```python
from build123d import *

# Parameters (mm, degrees)
SKETCH1_R               = 67.31
SKETCH1_R_2             = 54.61
BOSS_EXTRUDE1_DEPTH     = 57.15
CUT_EXTRUDE1_DEPTH      = 161.994729727
CUT_EXTRUDE1_DEPTH_BACK = 161.994729727
SKETCH2_R               = 1.2065
SKETCH3_R               = 1.2065
CUT_EXTRUDE2_DEPTH      = 171.985259226
CUT_EXTRUDE3_START      = -50.8
CUT_EXTRUDE3_DEPTH      = 50.8
SKETCH5_W               = 12.7
SKETCH5_H               = 152.473493429
CUT_EXTRUDE4_DEPTH      = 50.8
CUT_EXTRUDE5_START      = -19.05
CUT_EXTRUDE5_DEPTH      = 19.05
CUT_EXTRUDE6_START      = -19.05
CUT_EXTRUDE6_DEPTH      = 19.05
FILLET1_START           = 53
FILLET1_DEPTH           = 15
FILLET1_2_DEPTH         = 15
FILLET1_START_2         = -67.31
FILLET1_3_DEPTH         = 14.31
CUT_EXTRUDE7_START      = -19.05
CUT_EXTRUDE7_DEPTH      = 19.05


with BuildPart() as part:
    # Sketch1 → Boss-Extrude1 (new body)
    with BuildSketch(Plane(origin=(0, 0, 0), x_dir=(1, 0, 0), z_dir=(0, 1, 0))):
        with Locations(Location((0, 0, 0), (0, 0, 270))):
            Circle(SKETCH1_R)
        with Locations(Location((0, 0, 0), (0, 0, 270))):
            Circle(SKETCH1_R_2, mode=Mode.SUBTRACT)
    extrude(amount=BOSS_EXTRUDE1_DEPTH)

    # Sketch2 → Cut-Extrude1 (cut, two sides: drawn at the far end of the back side and taken through both)
    with BuildSketch(Plane.XY.offset(67.31).offset(-CUT_EXTRUDE1_DEPTH_BACK)):
        Polygon((-5.08, 51.435), (-6.35, 52.705), (-6.35, 50.165), align=None)
        Polygon((-6.35, 52.705), (-6.35, 57.15), (-19.05, 57.15), (-19.05, 25.0825), (-6.35, 25.0825), (-6.35, 50.165), align=None)
        Polygon((5.08, 51.435), (6.35, 50.165), (6.35, 52.705), align=None)
        Polygon((6.35, 50.165), (6.35, 25.0825), (19.05, 25.0825), (19.05, 57.15), (6.35, 57.15), (6.35, 52.705), align=None)
        with Locations((0, 51.435)):
            Circle(SKETCH2_R)
        with Locations((0, 28.575)):
            Circle(SKETCH2_R)
        with Locations((0, 5.715)):
            Circle(SKETCH2_R)
    extrude(amount=CUT_EXTRUDE1_DEPTH + CUT_EXTRUDE1_DEPTH_BACK, mode=Mode.SUBTRACT)

    # Sketch3 → Cut-Extrude2 (cut, through all)
    with BuildSketch(Plane(origin=(-58.292169929, 0, -33.655), x_dir=(0, -1, 0), z_dir=(-0.8660254037844364, 0, -0.5000000000000041))):
        with Locations(Location((-28.575, 0, 0), (0, 0, 90))):
            Circle(SKETCH3_R)
    cut_extrude2 = extrude(amount=-CUT_EXTRUDE2_DEPTH, mode=Mode.SUBTRACT)

    # Mirror1: Cut-Extrude2 across plane
    add(cut_extrude2.mirror(Plane(origin=(0, 0, 0), x_dir=(0, 0, 1), z_dir=(1, 0, 0))), mode=Mode.SUBTRACT)

    # Cut-Extrude3: read off the stored shape, not the designer's step
    # Cut-Extrude3 outline → Cut-Extrude3 (cut)
    with BuildSketch(Plane(origin=(0, 57.15, 0), x_dir=(1, 0, 0), z_dir=(0, 1, 0)).offset(CUT_EXTRUDE3_START)):
        with BuildLine():
            ThreePointArc((-6.35, -67.009802268), (0, -67.31), (6.35, -67.009802268))
            Line((6.35, -67.009802268), (-6.35, -67.009802268))
        make_face()
        with BuildLine():
            Line((6.35, -54.23955752), (6.35, -67.009802268))
            ThreePointArc((6.35, -67.009802268), (57.986556059, -34.178873833), (61.701920082, 26.898125551))
            Line((61.701920082, 26.898125551), (50.616947204, 20.498213476))
            ThreePointArc((50.616947204, 20.498213476), (46.986613751, -27.830023862), (6.35, -54.23955752))
        make_face()
        with BuildLine():
            Line((-6.35, -67.009802268), (-6.35, -54.23955752))
            ThreePointArc((-6.35, -54.23955752), (-46.986613751, -27.830023862), (-50.616947204, 20.498213476))
            Line((-50.616947204, 20.498213476), (-61.701920082, 26.898125551))
            ThreePointArc((-61.701920082, 26.898125551), (-57.986556059, -34.178873833), (-6.35, -67.009802268))
        make_face()
        with BuildLine():
            Line((54.145420082, 39.986367478), (61.701920082, 26.898125551))
            ThreePointArc((61.701920082, 26.898125551), (58.292169929, 33.655), (54.145420082, 39.986367478))
        make_face()
        with BuildLine():
            Line((-54.145420082, 39.986367478), (-43.060447204, 33.586455403))
            ThreePointArc((-43.060447204, 33.586455403), (0, 54.61), (43.060447204, 33.586455403))
            Line((43.060447204, 33.586455403), (54.145420082, 39.986367478))
            ThreePointArc((54.145420082, 39.986367478), (0, 67.31), (-54.145420082, 39.986367478))
        make_face()
    extrude(amount=CUT_EXTRUDE3_DEPTH, mode=Mode.SUBTRACT)

    # Sketch5 → Cut-Extrude4 (cut)
    with BuildSketch(Plane(origin=(0, 6.35, 0), x_dir=(1, 0, 0), z_dir=(0, 1, 0))):
        with Locations((0, 21.997189195)):
            Rectangle(SKETCH5_W, SKETCH5_H)
    extrude(amount=-CUT_EXTRUDE4_DEPTH, mode=Mode.SUBTRACT)

    # Sketch6 → Cut-Extrude5 (cut)
    with BuildSketch(Plane(origin=(0, 57.15, 0), x_dir=(1, 0, 0), z_dir=(0, 1, 0)).offset(CUT_EXTRUDE5_START)):
        with BuildLine():
            Line((50.616947204, 20.498213476), (61.701920082, 26.898125551))
            Line((61.701920082, 26.898125551), (54.145420082, 39.986367478))
            Line((54.145420082, 39.986367478), (43.060447204, 33.586455403))
            ThreePointArc((43.060447204, 33.586455403), (47.293647301, 27.305), (50.616947204, 20.498213476))
        make_face()
        with BuildLine():
            Line((-61.701920082, 26.898125551), (-50.616947204, 20.498213476))
            ThreePointArc((-50.616947204, 20.498213476), (-47.293647301, 27.305), (-43.060447204, 33.586455403))
            Line((-43.060447204, 33.586455403), (-54.145420082, 39.986367478))
            ThreePointArc((-54.145420082, 39.986367478), (-58.292169929, 33.655), (-61.701920082, 26.898125551))
        make_face()
    extrude(amount=CUT_EXTRUDE5_DEPTH, mode=Mode.SUBTRACT)

    # Sketch7 → Cut-Extrude6 (cut)
    with BuildSketch(Plane(origin=(0, 6.35, 0), x_dir=(1, 0, 0), z_dir=(0, 1, 0)).offset(CUT_EXTRUDE6_START)):
        with BuildLine():
            Line((6.35, 67.009802268), (6.35, 54.23955752))
            ThreePointArc((6.35, 54.23955752), (26.776589215, 47.594814528), (43.060447204, 33.586455403))
            Line((43.060447204, 33.586455403), (54.145420082, 39.986367478))
            ThreePointArc((54.145420082, 39.986367478), (33.128393708, 58.593051041), (6.35, 67.009802268))
        make_face()
        with BuildLine():
            Line((-6.35, 54.23955752), (-6.35, 67.009802268))
            ThreePointArc((-6.35, 67.009802268), (-33.128393708, 58.593051041), (-54.145420082, 39.986367478))
            Line((-54.145420082, 39.986367478), (-43.060447204, 33.586455403))
            ThreePointArc((-43.060447204, 33.586455403), (-26.776589215, 47.594814528), (-6.35, 54.23955752))
        make_face()
    extrude(amount=CUT_EXTRUDE6_DEPTH, mode=Mode.SUBTRACT)

    # Fillet1: read off the stored shape, not the designer's step
    # Fillet1 outline → Fillet1 (cut)
    with BuildSketch(Plane.XY.offset(FILLET1_START)):
        with BuildLine():
            Line((6.35, 57.15), (1.309843752, 57.15))
            ThreePointArc((1.309843752, 57.15), (4.669947917, 55.88), (6.35, 52.705))
            Line((6.35, 52.705), (6.35, 57.15))
        make_face()
        with BuildLine():
            ThreePointArc((-6.35, 52.705), (-4.669947917, 55.88), (-1.309843752, 57.15))
            Line((-1.309843752, 57.15), (-6.35, 57.15))
            Line((-6.35, 57.15), (-6.35, 52.705))
        make_face()
    extrude(amount=FILLET1_DEPTH, mode=Mode.SUBTRACT)

    # Fillet1 2 outline → Fillet1 2 (cut)
    with BuildSketch(Plane(origin=(0, 0, 0), x_dir=(0.5000000000000049, 0, 0.8660254037844358), z_dir=(0.8660254037844358, 0, -0.5000000000000049)).offset(FILLET1_START)):
        with BuildLine():
            Line((7.5565, -38.1), (7.5565, -33.02))
            ThreePointArc((7.5565, -33.02), (6.068602448, -36.612102448), (2.4765, -38.1))
            Line((2.4765, -38.1), (7.5565, -38.1))
        make_face()
        with BuildLine():
            Line((-7.5565, -38.1), (-2.4765, -38.1))
            ThreePointArc((-2.4765, -38.1), (-6.068602448, -36.612102448), (-7.5565, -33.02))
            Line((-7.5565, -33.02), (-7.5565, -38.1))
        make_face()
    extrude(amount=FILLET1_2_DEPTH, mode=Mode.SUBTRACT)

    # Fillet1 3 outline → Fillet1 3 (cut)
    with BuildSketch(Plane(origin=(0, 0, 0), x_dir=(0.49999999999999956, 0, -0.8660254037844389), z_dir=(0.8660254037844388, 0, 0.4999999999999999)).offset(FILLET1_START_2)):
        with BuildLine():
            Line((7.5565, 38.1), (2.4765, 38.1))
            ThreePointArc((2.4765, 38.1), (6.068602448, 36.612102448), (7.5565, 33.02))
            Line((7.5565, 33.02), (7.5565, 38.1))
        make_face()
        with BuildLine():
            ThreePointArc((-7.5565, 33.02), (-6.068602448, 36.612102448), (-2.4765, 38.1))
            Line((-2.4765, 38.1), (-7.5565, 38.1))
            Line((-7.5565, 38.1), (-7.5565, 33.02))
        make_face()
    extrude(amount=FILLET1_3_DEPTH, mode=Mode.SUBTRACT)

    # Sketch8 → Cut-Extrude7 (cut)
    with BuildSketch(Plane(origin=(0, 6.35, 0), x_dir=(1, 0, 0), z_dir=(0, 1, 0)).offset(CUT_EXTRUDE7_START)):
        with BuildLine():
            ThreePointArc((-6.35, -67.009802268), (-3.690833292, -67.208733433), (-1.025873896, -67.302181857))
            Line((-1.025873896, -67.302181857), (-1.025873896, -67.009802268))
            Line((-1.025873896, -67.009802268), (-6.35, -67.009802268))
        make_face()
        Polygon((-1.025873896, -67.009802268), (-1.025873896, -67.302181857), (-1.551971907, -68.232150278), (0.972160244, -68.180468419), (1.025873896, -67.302181857), (1.025873896, -67.009802268), align=None)
        with BuildLine():
            Line((6.35, -67.009802268), (1.025873896, -67.009802268))
            Line((1.025873896, -67.009802268), (1.025873896, -67.302181857))
            ThreePointArc((1.025873896, -67.302181857), (3.690833292, -67.208733433), (6.35, -67.009802268))
        make_face()
        with BuildLine():
            ThreePointArc((61.701920082, 26.898125551), (58.292169929, 33.655), (54.145420082, 39.986367478))
            Line((54.145420082, 39.986367478), (61.701920082, 26.898125551))
        make_face()
    extrude(amount=CUT_EXTRUDE7_DEPTH, mode=Mode.SUBTRACT)


solid = part.part
```
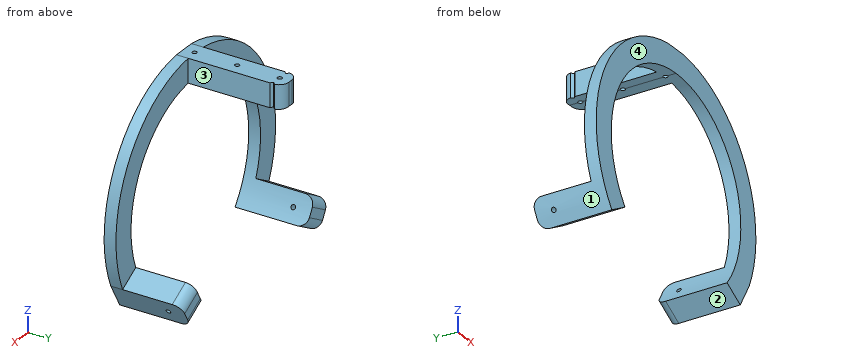
Here's how the part is built. I have some questions about the finished solid (model axes, mm). Face numbers are marked on the shaded views. Coordinates: 2 decimals unless noted, no trailing zeros. Order: outer loops, then holes, each group sorted by start corner. A loop starts at its lowest first (then second) coordinate and runs counter-clockwise, first axis right, second up. Notation, with made-up numbers: (68, 42) -> (106, 42) arc R13 ccw to (106, 52) -> close; hole circle Ø6 at (-24.75, 78). An arc over 180 degrees is marked (long way). Return JSON: item names as keys, results as strings.
1) If we section it at A-A on y = 15: List the corners of the cut face in (x, z) for me.
Conclusion:
{"outline": "(-61.7, -26.9) arc R67.31 ccw to (-54.15, -39.99) -> (-43.06, -33.59) arc R54.61 cw to (-50.62, -20.5) -> close; (-6.35, 54.24) arc R54.61 cw to (6.35, 54.24) -> (6.35, 67.01) -> (-6.35, 67.01) -> close; (43.06, -33.59) -> (54.15, -39.99) -> (61.7, -26.9) -> (50.62, -20.5) arc R54.61 cw to start"}
2) If I drill on probe 1 along Y at (x, z) = (0, 61.5); probe 2 along X at (y, z) = (2, 1.5); probe 3 along X at (y, z) = (51.5, 56.5) (3 decimals), over which ranges is the centre line in solid material (lowest first)?
Conclusion:
{"probe 1": "y = 0 to 4.51, 6.92 to 27.37, 29.78 to 50.23, 52.64 to 57.15", "probe 2": "x = -67.29 to -54.59, 54.59 to 67.29", "probe 3": "x = -5.145 to -1.205, 1.205 to 5.145"}
3) If we section it at C-C on z = 41: List the corners of the cut face in (x, y) for me.
Conclusion:
{"outline": "(-53.38, 0) -> (-36.07, 0) -> (-36.07, 6.35) -> (-53.38, 6.35) -> close; (36.07, 0) -> (53.38, 0) -> (53.38, 6.35) -> (36.07, 6.35) -> close"}
4) If we section it at D-D on y = 42: List the corners of the cut face in (x, z) for me, plus the area to 3 significant figures.
Conclusion:
{"outline": "(-6.35, 54.24) arc R54.61 cw to (6.35, 54.24) -> (6.35, 67.01) -> (-6.35, 67.01) -> close", "area": "159 mm²"}
5) If we section it at B-B on z = -7.5: List the corners of the cut face in (x, y) for me.
Conclusion:
{"outline": "(-66.89, 0) -> (-54.09, 0) -> (-54.09, 6.35) -> (-66.89, 6.35) -> close; (54.09, 0) -> (66.89, 0) -> (66.89, 6.35) -> (54.09, 6.35) -> close"}
6) I'm going to push flat-ended pins straight in: P1, Ø5, axis at x = 53, z = -28.5, coming from the +Y side; P2, Ø1.4, axis at x = 0, y = 51.435, coming from the -Z side; P3, Ø10, axis at y = 18.5, z = 59.5, coming from the -X side; P4, Ø12, axis at x = 38.5, y = 6, coming from the -Z side. Where does each tip first touch, or does it pass through?
Conclusion:
{"P1": "stops at y = 38.1", "P2": "passes through", "P3": "stops at x = -6.35", "P4": "stops at z = -34.42"}
7) Thinking about a two-plate mould opening in X: for the marked faces 1, 2, 3 and 4, which applies, +X half, -X half, draft (parallel to the pull), parting line (faces both ways), or undercut?
Conclusion:
{"face 1": "-X half", "face 2": "undercut", "face 3": "+X half", "face 4": "draft"}
